Input: part model. Units: mm. Frame: model coordinates. Round coordinates to 2 decimals unless told otherwise and drop trailing zeros. Loops run counter-clockwise (first coordinate to the right, second up) from the corner with the lowest first, then second, coordinate; pieces in that order, holes last. Notation, with made-up numbers: (24, -8.75) - (54, -8.75) arc R4 ccw to (54, -4.75) - close; hole circle Ø3 at (46, 31). An arc over 180 degrees is marked (long way). Use CSV: the item, a comma, the result in double quotes. Start each with the question number.
1. Material intervals for probe 1 along X at (y, z) = (49.5, 0); probe 2 along Y at (x, z) = (94, 0); probe 3 along Z at (x, y) = (-40, 17), sorted ascending. Write a range as from..to.
2. Cut plane C-C (y = 65). Return loops of the section in (x, z).
3. Pull-direction query (Z, two-part tool) for faces 1 (the cylindrical face through (66.378, 39.674, 66.67)), 2 (the cylindrical face through (61.82, 37.57, 80.63)), 3 (the cylindrical face through (-65.921, 39.439, 67.128)), 4 (the flat face through (75, 0, 46)); classes: +Z half, -Z half, draft (parallel to the pull), parting line (faces both ways), or undercut.
4. Pin query (flat end, axial travel): P1, Ø5, axis at y = 52, z = -50.5, coming from the +X side; P2, Ø6, axis at y = 19.5, z = 70.5, coming from the -X side; P3, Ø4, axis at y = 55, z = -53.5, coming from the +X side. Return the tip coordinate at first contact, or that it passes through.
5. Cut plane A-A (x = -9.5). Return loops of the section in (y, z).
6. Cut plane B-B (z = -30). Return loops of the section in (x, y).
```python
from build123d import *

# Parameters (mm, degrees)
SKETCH1_R               = 101.6
SKETCH1_R_2             = 86.36
BOSS_EXTRUDE1_DEPTH     = 76.2
CUT_EXTRUDE1_REACH      = 241.623
CUT_EXTRUDE1_END_RADIUS = 86.36
SKETCH2_R               = 1.5875
CIRPATTERN1_COUNT       = 8


with BuildPart() as part:
    # Sketch1 → Boss-Extrude1 (new body)
    with BuildSketch(Plane(origin=(0, 0, 0), x_dir=(1, 0, 0), z_dir=(0, 1, 0))):
        with Locations(Location((0, 0, 0), (0, 0, 90))):
            Circle(SKETCH1_R)
        with Locations(Location((0, 0, 0), (0, 0, 90))):
            Circle(SKETCH1_R_2, mode=Mode.SUBTRACT)
    extrude(amount=BOSS_EXTRUDE1_DEPTH)

    # Cut-Extrude1: up to this cylinder (the profile starts outside it)
    cut_extrude1_end = Plane(origin=(0, 38.1, 0), z_dir=(0, -1, 0)) * Cylinder(CUT_EXTRUDE1_END_RADIUS, 656.966, mode=Mode.PRIVATE)
    # Sketch2 → Cut-Extrude1 (cut, up to the surface)
    with BuildSketch(Plane.XY.offset(101.6), mode=Mode.PRIVATE) as cut_extrude1_sk1:
        with Locations((0, 38.1)):
            Circle(SKETCH2_R)
    cut_extrude1_tool1 = extrude(cut_extrude1_sk1.sketch, amount=-CUT_EXTRUDE1_REACH, mode=Mode.PRIVATE) - cut_extrude1_end
    cut_extrude1 = cut_extrude1_tool1.solids().sort_by_distance((0, 38.1, 101.6))[0]
    add(cut_extrude1, mode=Mode.SUBTRACT)

    # CirPattern1: Cut-Extrude1 ×8 about axis
    cirpattern1_axis = Axis((0, 76.2, 0), (0, -1, 0))
    for i in range(1, CIRPATTERN1_COUNT):
        add(cut_extrude1.rotate(cirpattern1_axis, i * 360 / CIRPATTERN1_COUNT), mode=Mode.SUBTRACT)


solid = part.part
```
Established:
1,probe 1,"x = -101.6..-86.36, 86.36..101.6"
1,probe 2,"y = 0..36.51, 39.69..76.2"
1,probe 3,"z = -93.39..-76.54, 76.54..93.39"
2,outline,"circle Ø203.2 at (0, 0); hole circle Ø172.72 at (0, 0)"
3,face 1,"undercut"
3,face 2,"parting line"
3,face 3,"undercut"
3,face 4,"draft"
4,P1,"stops at x = 89.55"
4,P2,"stops at x = -75.94"
4,P3,"stops at x = 87.58"
5,outline,"(0, -101.15) - (76.2, -101.15) - (76.2, -85.84) - (0, -85.84) - close; (0, 85.84) - (76.2, 85.84) - (76.2, 101.15) - (0, 101.15) - close"
6,outline,"(-97.07, 0) - (-80.98, 0) - (-80.98, 76.2) - (-97.07, 76.2) - close; (80.98, 0) - (97.07, 0) - (97.07, 76.2) - (80.98, 76.2) - close"
